from build123d import *

# Parameters (mm, degrees)
F2_DEPTH = 25.4


with BuildPart() as f2:
    # F1 (on face) → F2 (new body)
    with BuildSketch(Plane.XY):
        with BuildLine():
            ThreePointArc((-4.8808341445, 14.0525419265), (-5.004069886, 14.0091313477), (-5.1269195974, 13.9646400592))
            Line((-5.1269195974, 13.9646400592), (-5.1269195974, 1.288408295))
            ThreePointArc((-5.1269195974, 1.288408295), (-1.4388144753, 5.0867586338), (3.6924446467, 3.783008462))
            Line((3.6924446467, 3.783008462), (3.6924446467, 14.4104937137))
            ThreePointArc((3.6924446467, 14.4104937137), (3.6125240495, 14.4307361744), (3.5324924947, 14.450535399))
            Line((3.5324924947, 14.450535399), (3.0549003277, 14.0525419265))
            Line((3.0549003277, 14.0525419265), (-4.8808341445, 14.0525419265))
        make_face()
        with BuildLine():
            Line((-5.1269195974, 1.288408295), (-5.1269195974, 13.9646400592))
            ThreePointArc((-5.1269195974, 13.9646400592), (-8.5155220323, -12.1976375196), (14.8760369905, 0))
            ThreePointArc((14.8760369905, 0), (11.752136395, 9.1205135105), (3.6924446467, 14.4104937137))
            Line((3.6924446467, 14.4104937137), (3.6924446467, 3.783008462))
            ThreePointArc((3.6924446467, 3.783008462), (4.8715904415, 2.0525367386), (5.2863314778, 0))
            ThreePointArc((5.2863314778, 0), (4.8715904415, -2.0525367386), (3.6924446467, -3.783008462))
            Line((3.6924446467, -3.783008462), (3.6924446467, -11.555492878))
            Line((3.6924446467, -11.555492878), (-4.7550187446, -10.9179485589))
            Line((-4.7550187446, -10.9179485589), (-5.1269195974, -10.9179485589))
            Line((-5.1269195974, -10.9179485589), (-5.1269195974, -1.288408295))
            ThreePointArc((-5.1269195974, -1.288408295), (-5.2863314778, 0), (-5.1269195974, 1.288408295))
        make_face()
        with BuildLine():
            ThreePointArc((3.5324924947, 14.450535399), (-0.7029267403, 14.8594202626), (-4.8808341445, 14.0525419265))
            Line((-4.8808341445, 14.0525419265), (3.0549003277, 14.0525419265))
            Line((3.0549003277, 14.0525419265), (3.5324924947, 14.450535399))
        make_face()
        with BuildLine():
            ThreePointArc((3.6924446467, -3.783008462), (-1.4388144753, -5.0867586338), (-5.1269195974, -1.288408295))
            Line((-5.1269195974, -1.288408295), (-5.1269195974, -10.9179485589))
            Line((-5.1269195974, -10.9179485589), (-4.7550187446, -10.9179485589))
            Line((-4.7550187446, -10.9179485589), (3.6924446467, -11.555492878))
            Line((3.6924446467, -11.555492878), (3.6924446467, -3.783008462))
        make_face()
    extrude(amount=F2_DEPTH)


solid = f2.part
Verification items for the finished model (mm, model axes). Round coordinates to 2 decimals unless told otherwise and drop trailing zeros. Write each loop counter-clockwise with the first axis right and the second up, starting at its lowest first coordinate (ties: lowest second). Pieces come first, ordered by that corner, then holes.
(1) Material ranges on line 1 (Y direction, x = 1.25, z = 20.25); line 2 (Y direction, x = 4.5, z = 3.75), recorded low to high.
Returned:
line 1: y = -14.82 to -5.14, 5.14 to 14.82
line 2: y = -14.18 to -2.77, 2.77 to 14.18
(2) Section check C-C (y = -4.5). Enter the section's corners in (x, z).
Returned:
outline: (-14.18, 0) - (-2.77, 0) - (-2.77, 25.4) - (-14.18, 25.4) - close; (2.77, 0) - (14.18, 0) - (14.18, 25.4) - (2.77, 25.4) - close
(3) Section check A-A (x = 0). Enter the section's corners in (y, z), plus the area to 3 significant figures.
Returned:
outline: (-14.88, 0) - (-5.29, 0) - (-5.29, 25.4) - (-14.88, 25.4) - close; (5.29, 0) - (14.88, 0) - (14.88, 25.4) - (5.29, 25.4) - close
area: 487 mm2
(4) Depth check by flat-ended pin: pin 1 Ø3 at (y, z) = (-1, 15) entering from +X; pin 2 Ø6 at (x, z) = (5.5, 17.5) entering from -Y; pin 3 Ø5 at (x, z) = (8.5, 22.5) entering from +Y. Enter the tip coordinate at first touch or a pass-through.
Returned:
pin 1: stops at x = 14.88
pin 2: stops at y = -14.66
pin 3: stops at y = 13.61
(5) Section check B-B (z = 20). Enter the section's corners in (x, y).
Returned:
outline: (3.53, 14.45) arc R14.88 ccw (long way) to (3.69, 14.41) arc R14.88 ccw to start; hole circle Ø10.57 at (0, 0)
(6) Section check D-D (x = -10.25). Enter the section's corners in (y, z).
Returned:
outline: (-10.78, 0) - (10.78, 0) - (10.78, 25.4) - (-10.78, 25.4) - close
